```python
from build123d import *

# Parameters (mm, degrees)
SKETCH2_W             = 20
SKETCH2_H             = 20
BOSS_EXTRUDE1_DEPTH   = 30
BOSS_EXTRUDE1_2_DEPTH = 30
SKETCH3_W             = 16
SKETCH3_H             = 16
CUT_EXTRUDE1_DEPTH    = 26
SKETCH4_R             = 3
CUT_EXTRUDE2_DEPTH    = 56
SKETCH7_W             = 20
SKETCH7_H             = 4
BOSS_EXTRUDE2_DEPTH   = 160
CUT_EXTRUDE5_DEPTH    = 140
SKETCH10_W            = 1
SKETCH10_H            = 37.358544319
CUT_EXTRUDE6_DEPTH    = 140


with BuildPart() as part:
    # Sketch2 → Boss-Extrude1 (new body)
    with BuildSketch(Plane(origin=(0, 0, 0), x_dir=(1, 0, 0), z_dir=(0, 1, 0))):
        with Locations((10, 10)):
            Rectangle(SKETCH2_W, SKETCH2_H)
    extrude(amount=BOSS_EXTRUDE1_DEPTH)


with BuildPart() as body_2:
    # Sketch2 → Boss-Extrude1 2 (new body)
    with BuildSketch(Plane(origin=(0, 0, 0), x_dir=(1, 0, 0), z_dir=(0, 1, 0))):
        with Locations((10, -170)):
            Rectangle(SKETCH2_W, SKETCH2_H)
    extrude(amount=BOSS_EXTRUDE1_2_DEPTH)


with BuildPart() as cut_extrude1_tool:
    # Sketch3 → Cut-Extrude1 (new body)
    with BuildSketch(Plane(origin=(0, 30, 0), x_dir=(1, 0, 0), z_dir=(0, 1, 0))):
        with Locations((10, 10)):
            Rectangle(SKETCH3_W, SKETCH3_H)
        with Locations((10, -170)):
            Rectangle(SKETCH3_W, SKETCH3_H)
    extrude(amount=-CUT_EXTRUDE1_DEPTH)


with BuildPart() as part_1:
    add(part.part)

    # Cut-Extrude1: cut by cut_extrude1_tool
    add(cut_extrude1_tool.part, mode=Mode.SUBTRACT)


with BuildPart() as body_2_1:
    add(body_2.part)

    # Cut-Extrude1: cut by cut_extrude1_tool
    add(cut_extrude1_tool.part, mode=Mode.SUBTRACT)


with BuildPart() as cut_extrude2_tool:
    # Sketch4 → Cut-Extrude2 (new body)
    with BuildSketch(Plane(origin=(0, 4, 0), x_dir=(1, 0, 0), z_dir=(0, 1, 0))):
        with Locations(Location((10, -170, 0), (0, 0, 270))):
            Circle(SKETCH4_R)
        with Locations(Location((10, 10, 0), (0, 0, 270))):
            Circle(SKETCH4_R)
    extrude(amount=-CUT_EXTRUDE2_DEPTH)


with BuildPart() as part_2:
    add(part_1.part)

    # Cut-Extrude2: cut by cut_extrude2_tool
    add(cut_extrude2_tool.part, mode=Mode.SUBTRACT)



with BuildPart() as body_2_2:
    add(body_2_1.part)

    # Cut-Extrude2: cut by cut_extrude2_tool
    add(cut_extrude2_tool.part, mode=Mode.SUBTRACT)


with BuildPart() as part_3:
    add(part_2.part)

    add(body_2_2.part)  # Boss-Extrude2 merges body 2
    # Sketch7 → Boss-Extrude2 (add)
    with BuildSketch(Plane(origin=(0, 0, 160), x_dir=(-1, 0, 0), z_dir=(0, 0, -1))):
        with Locations((-10, 28)):
            Rectangle(SKETCH7_W, SKETCH7_H)
    extrude(amount=BOSS_EXTRUDE2_DEPTH)

    # Sketch9 → Cut-Extrude5 (cut)
    with BuildSketch(Plane(origin=(20, 0, 0), x_dir=(0, 0, -1), z_dir=(1, 0, 0))):
        Polygon((-180, 15), (-165, 30), (-180, 30), align=None)
        Polygon((20, 15), (5, 30), (20, 30), align=None)
    extrude(amount=-CUT_EXTRUDE5_DEPTH, mode=Mode.SUBTRACT)

    # Sketch10 → Cut-Extrude6 (cut)
    with BuildSketch(Plane(origin=(20, 0, 0), x_dir=(0, 0, -1), z_dir=(1, 0, 0))):
        with Locations((-179.5, 18.67927216)):
            Rectangle(SKETCH10_W, SKETCH10_H)
        with Locations((19.5, 18.67927216)):
            Rectangle(SKETCH10_W, SKETCH10_H)
    extrude(amount=-CUT_EXTRUDE6_DEPTH, mode=Mode.SUBTRACT)


solid = part_3.part
```
Verification items for the finished model (mm, model axes). A direction names the side the tool comes from. Coordinates: 2 decimals unless noted, no trailing zeros. Loops run counter-clockwise (first coordinate to the right, second up) from the corner with the lowest first, then second, coordinate; pieces in that order, holes last. Notation, with made-up numbers: (28, 17) -> (46, 17) arc R29 ccw to (46, 53) -> close; hole circle Ø7 at (35, 80). An arc over 180 degrees is marked (long way). Put each result on its own line as item: value.
1. Section check B-B, the plane z = 170. Record the boundary of the cut face in (x, y).
Result set:
outline: (0, 0) -> (7, 0) -> (7, 4) -> (2, 4) -> (2, 25) -> (0, 25) -> close; (13, 0) -> (20, 0) -> (20, 25) -> (18, 25) -> (18, 4) -> (13, 4) -> close
2. Gauge pin test, flat ends, axial feed: P1, Ø1, axis at x = 6, z = 31.5, coming from the -Y side; P2, Ø5, axis at x = 16, y = 23.5, coming from the -Z side; P3, Ø5, axis at x = 13, y = 20, coming from the +Z side. Record the tip position at first contact, or that the pin passes through.
Result set:
P1: stops at y = 26
P2: stops at z = -13
P3: stops at z = 162
3. Section check A-A, the plane y = 5.75. Record the boundary of the cut face in (x, z).
Result set:
outline: (0, -19) -> (20, -19) -> (20, 0) -> (0, 0) -> close; (0, 160) -> (20, 160) -> (20, 179) -> (0, 179) -> close; hole (2, -18) -> (18, -18) -> (18, -2) -> (2, -2) -> close; hole (2, 162) -> (18, 162) -> (18, 178) -> (2, 178) -> close
4. Thickness scan on line 1 (Z direction, x = 8, y = 11.25); line 2 (Z direction, x = 8.75, y = 25.25); line 3 (X direction, y = 1.25, z = -10). Record the ranges inside material, lowest first.
Result set:
line 1: z = -19 to -18, -2 to 0, 160 to 162, 178 to 179
line 2: z = -2 to 0, 160 to 162
line 3: x = 0 to 7, 13 to 20
5. Section check D-D, the plane z = 77. Record the boundary of the cut face in (x, y), then the cut area to 3 significant figures.
Result set:
outline: (0, 26) -> (20, 26) -> (20, 30) -> (0, 30) -> close
area: 80.0 mm^2
6. Mould release check, pull along X, two halves, no side actions. Record for faces 4 (the face through (2, 14, -8)), 5 (the face through (0, 27, 73)), 6 (the face through (12, 0, 167)), 7 (the face through (20, 27, 73)): pulls with the +X half, pulls with the -X half, needs draft (parallel to the pull), parting line crosses it, or undercut.
Result set:
face 4: undercut
face 5: pulls with the -X half
face 6: needs draft
face 7: pulls with the +X half
7. Tool access check on faces 1 (the face through (10, 13, 160)), 2 (the face through (9.9, 4, 173.4)), 3 (the face through (10, 30, 81)). Record the directions out of +Z, -Z, +X, -X, +Y, -Y that give a thin tool (end or side, any length) a straight path to the whole face; none if there is none.
Result set:
face 1: +X, -X, -Y
face 2: +Y
face 3: +Z, -Z, +X, -X, +Y
8. Section check C-C, the plane x = 10. Record the boundary of the cut face in (y, z).
Result set:
outline: (0, -19) -> (16, -19) -> (17, -18) -> (4, -18) -> (4, -13) -> (0, -13) -> close; (0, -7) -> (4, -7) -> (4, -2) -> (30, -2) -> (30, 162) -> (4, 162) -> (4, 167) -> (0, 167) -> (0, 160) -> (26, 160) -> (26, 0) -> (0, 0) -> close; (0, 173) -> (4, 173) -> (4, 178) -> (17, 178) -> (16, 179) -> (0, 179) -> close
